Geometry check sheet. Reference: the model listing, model coordinates, mm. A direction names the side the tool comes from. Give positions to 0.01 mm unless a question says otherwise; leave off trailing zeros. Loops run counter-clockwise (first coordinate to the right, second up) from the corner with the lowest first, then second, coordinate; pieces in that order, holes last. Notation, with made-up numbers: (50, 42) - (103, 42) arc R17 ccw to (103, 65) - close; hole circle Ø6 at (25, 77.25). An arc over 180 degrees is marked (long way). One line per question, with ' | ' between items. Start each with the question number.
Autodesk Inventor part; units mm, degrees
ref_plane "YZ Plane" through (0, 0, 0) normal (1, 0, 0) x (0, 1, 0)
ref_plane "XZ Plane" through (0, 0, 0) normal (0, 1, 0) x (-1, 0, 0)
ref_plane "XY Plane" through (0, 0, 0) normal (0, 0, 1) x (1, 0, 0)
sketch "Sketch1" plane through (0, 0, 0) normal (0, 1, 0) x (-1, 0, 0)
  line L0 (0, 0) -> (31.75, 0)
  line L1 (31.75, 0) -> (31.75, -114.3)
  line L2 (31.75, -114.3) -> (0, -114.3)
  line L3 (0, -114.3) -> (0, 0)
  dimension "d0" = 31.75
  dimension "d1" = 114.3
extrude "Extrusion1" add sketch "Sketch1" along normal blind 31.75
shell "Shell1" thickness 1.905 removed faces 3 at (-10.5833, 10.5833, 0) at (-21.1667, 21.1667, -114.3) at (-10.5833, 31.75, -38.1)
sketch "Sketch2" plane through (-31.75, 0, 0) normal (0, 0, 1) x (1, 0, 0)
  line L0 (1.905, 1.905) -> (1.905, 31.75)
  line L1 (29.845, 31.75) -> (29.845, 1.905)
  line L2 (1.905, 31.75) -> (5.715, 31.75)
  line L3 (5.715, 31.75) -> (1.905, 21.8784)
  line L4 (1.905, 31.75) -> (1.905, 1.905)
  line L5 (29.845, 31.75) -> (26.035, 31.75)
  line L6 (26.035, 31.75) -> (29.845, 21.8784)
  point P0 (31.75, 0)
  dimension "d5" = 3.81
extrude "Extrusion2" add sketch "Sketch2" against normal up to surface (114.3 mm away)
sketch "Sketch4" plane through (-31.75, 0, 0) normal (0, 0, 1) x (1, 0, 0)
  line L0 (1.905, 21.8784) -> (5.715, 31.75)
  line L1 (29.845, 21.8784) -> (26.035, 31.75)
  line L2 (5.715, 31.75) -> (26.035, 31.75)
  line L3 (1.905, 21.8784) -> (29.845, 21.8784)
  point P0 (31.75, 0)
extrude "Extrusion3" add sketch "Sketch4" against normal blind 6.35
sketch "Sketch5" plane through (0, 0, -114.3) normal (0, 0, -1) x (-1, 0, 0)
  line L0 (26.035, 31.75) -> (29.845, 21.8784)
  line L1 (26.035, 31.75) -> (5.715, 31.75)
  line L2 (1.905, 21.8784) -> (5.715, 31.75)
  line L3 (1.905, 21.8784) -> (29.845, 21.8784)
  point P0 (0, 0)
extrude "Extrusion4" add sketch "Sketch5" against normal blind 6.35
properties part number "MidshipsUnibody"
(1) Section check A-A, the plane y = 12.5. Record the boundary of the cut face in (x, z) (3 decimals), and give its area (3 significant figures).
(2) Depth check by flat-ended pin: pin 1 Ø8.5 at (x, z) = (-21, -81.5) entering from +Y (3 decimals). Enter the tip coordinate at first touch or a pass-through.
(3) Section check D-D, the plane x = -4. Record the boundary of the cut face in (y, z) (3 decimals), and give its area (3 significant figures).
(4) Material ranges on line 1 (X direction, y = 13, z = -71.5) (3 decimals); line 2 (Z direction, x = -16.5, y = 30.5); line 3 (Y direction, x = -11.5, z = -99.5) (3 decimals), recorded low to high.
(5) Section check C-C, the plane z = -105. Record the boundary of the cut face in (x, y) (3 decimals), and give its area (3 significant figures).
(6) Section check B-B, the plane x = -9. Record the boundary of the cut face in (y, z) (3 decimals).
(7) Tool access check on faces 1 (the face through (-31.75, 16, -56)), 2 (the face through (-27.913, 26.883, -56.439)), 3 (the face through (-1.905, 12, -58)). Record the directions out of +Z, -Z, +X, -X, +Y, -Y that give a thin tool (end or side, any length) a straight path to the whole face; none if there is none.
(8) Mould release check, pull along Z, two halves, no side actions. Record for faces 4 (the face through (-16, 0, -56)), 5 (the face through (-20, 23, 0)), 6 (the face through (-16, 27, -107.95)): pulls with the +Z half, pulls with the -Z half, needs draft (parallel to the pull), parting line crosses it, or undercut.
Numbers:
1) outline: (-31.75, -114.3) - (-29.845, -114.3) - (-29.845, 0) - (-31.75, 0) - close; (-1.905, -114.3) - (0, -114.3) - (0, 0) - (-1.905, 0) - close | area: 435 mm^2
2) pin 1: y = 1.905
3) outline: (0, -114.3) - (1.905, -114.3) - (1.905, 0) - (0, 0) - close; (21.878, -114.3) - (31.75, -114.3) - (31.75, 0) - (21.878, 0) - (21.878, -6.35) - (27.306, -6.35) - (27.306, -107.95) - (21.878, -107.95) - close | area: 795 mm^2
4) line 1: -31.75 to -29.845, -1.905 to 0 | line 2: -114.3 to -107.95, -6.35 to 0 | line 3: 0 to 1.905
5) outline: (-31.75, 0) - (0, 0) - (0, 31.75) - (-5.715, 31.75) - (-1.905, 21.878) - (-1.905, 1.905) - (-29.845, 1.905) - (-29.845, 21.878) - (-26.035, 31.75) - (-31.75, 31.75) - close | area: 212 mm^2
6) outline: (0, -114.3) - (1.905, -114.3) - (1.905, 0) - (0, 0) - close; (21.878, -114.3) - (31.75, -114.3) - (31.75, -107.95) - (21.878, -107.95) - close; (21.878, -6.35) - (31.75, -6.35) - (31.75, 0) - (21.878, 0) - close
7) face 1: +Z, -Z, -X, +Y, -Y | face 2: none | face 3: +Z, -Z
8) face 4: needs draft | face 5: pulls with the +Z half | face 6: undercut
